Geometry: final body of the model. Coordinates: model frame, mm. Face numbers are marked on the shaded views. A direction names the side the tool comes from. Give positions to 0.01 mm unless a question says otherwise; leave off trailing zeros. Write each loop counter-clockwise with the first axis right and the second up, starting at its lowest first coordinate (ties: lowest second). Pieces come first, ordered by that corner, then holes. Notation, with made-up numbers: M 23.25,31.5 L 41.25,31.5 A15 ccw 41.25,44.5 Z; hole C 21.25,-1.5 d5. An arc over 180 degrees is marked long. Use one line per item in the form item = value. Start each with the question number.
Item 1: Section query C-C on x = -8. Return loops of the section in (y, z).
Item 2: Access query for the marked faces 1 and 2. Directions: +Z, -Z, +X, -X, +Y, -Y. A direction counts if a zero-diameter tool reaches every point of the face in a straight line with its end or side. Return the directions, or none.
Item 3: Contact query for flat-ended pins moving along their axis: P1, Ø5, axis at x = -22, z = -3.5, coming from the +Y side; P2, Ø4, axis at y = -7, z = 5, coming from the +X side; P3, Ø12, axis at x = -22, y = -8.5, coming from the -Z side. Output: stop coordinate, or through.
Item 4: Section query D-D on x = 10. Return loops of the section in (y, z).
Item 5: Section query A-A on y = 0. Return loops of the section in (x, z), then the cut area to 4 significant figures.
Item 6: Material intervals for line 1 along Z through (x, y) = (-6, -6); line 2 along X through (y, z) = (0.5, 9.5); line 3 along Z through (x, y) = (-7.5, 0.25), sorted ascending. Write a range as from..to.
Item 7: Section query B-B on z = 5.75. Return loops of the section in (x, y), then the cut area to 3 significant figures.
from build123d import *

# Parameters (mm, degrees)
TROU_TARAUD_M3X0_51_D           = 2.5
TROU_TARAUD_M3X0_51_DEPTH       = 8.5
TROU_TARAUD_M3X0_51_CSINK_D     = 3.05
TROU_TARAUD_M3X0_51_CSINK_ANGLE = 90
TROU_TARAUD_M3X0_51_TIP         = 0.751075774


with BuildPart() as part:
    # Esquisse1 → Révolution1 (revolve)
    with BuildSketch(Plane.XY):
        Polygon((15.5, 2.5), (15.5, 0), (-27, 0), (-27, 15), (0, 15), (0, 8), (3, 8), (3, 2.5), align=None)
    revolve(axis=Axis((-51.155053474, 0, 0), (1, 0, 0)))

    # Trou taraudé M3x0.51
    with Locations(Plane(origin=(0, 0, 0), x_dir=(0, 0, -1), z_dir=(1, 0, 0))):
        with Locations((0, 12), (-10.392304845, -6), (10.392304845, -6)):
            CounterSinkHole(TROU_TARAUD_M3X0_51_D / 2, TROU_TARAUD_M3X0_51_CSINK_D / 2, depth=TROU_TARAUD_M3X0_51_DEPTH, counter_sink_angle=TROU_TARAUD_M3X0_51_CSINK_ANGLE)
            with Locations((0, 0, -(TROU_TARAUD_M3X0_51_DEPTH + TROU_TARAUD_M3X0_51_TIP / 2))):  # 118° drill point
                Cone(0, TROU_TARAUD_M3X0_51_D / 2, TROU_TARAUD_M3X0_51_TIP, mode=Mode.SUBTRACT)


solid = part.part
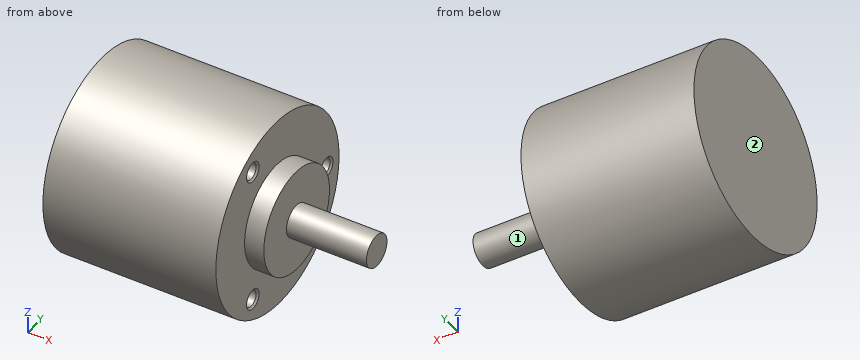
Answer sheet:
q1.outline = C 0,0 d30; hole C -6,-10.39 d2.5; hole C -6,10.39 d2.5; hole C 12,0 d2.5
q2.face_1 = +X
q2.face_2 = +Z, -Z, -X, +Y, -Y
q3.P1 = 14.97
q3.P2 = 3
q3.P3 = -14.79
q4.outline = C 0,0 d5
q5.outline = M -27,-15 L 0,-15 L 0,-8 L 3,-8 L 3,-2.5 L 15.5,-2.5 L 15.5,2.5 L 3,2.5 L 3,8 L 0,8 L 0,15 L -27,15 Z
q5.area = 920.5 mm2
q6.line_1 = -13.75..-11.64, -9.14..9.14, 11.64..13.75
q6.line_2 = -27..0
q6.line_3 = -15..15
q7.outline = M -27,-13.85 L 0,-13.85 L 0,-5.56 L 3,-5.56 L 3,5.56 L 0,5.56 L 0,13.85 L -27,13.85 Z
q7.area = 781 mm2
